Can you work these out from the drawing? Everything is in mm from the part's minimum corner. Give positions to 0.01 mm unless a question says otherwise; leave off trailing zeros. Loops run counter-clockwise (first coordinate to the right, second up) from the corner with the lowest first, then second, coordinate; pieces in that order, holes last. Notation, with made-up numbers: (-10.5, 60) - (9.5, 60) arc R30 cw to (9.5, 87) - close; hole circle Ø10 at (4, -7). An arc over 180 degrees is marked (long way). Answer in a Markdown table with one row per item.
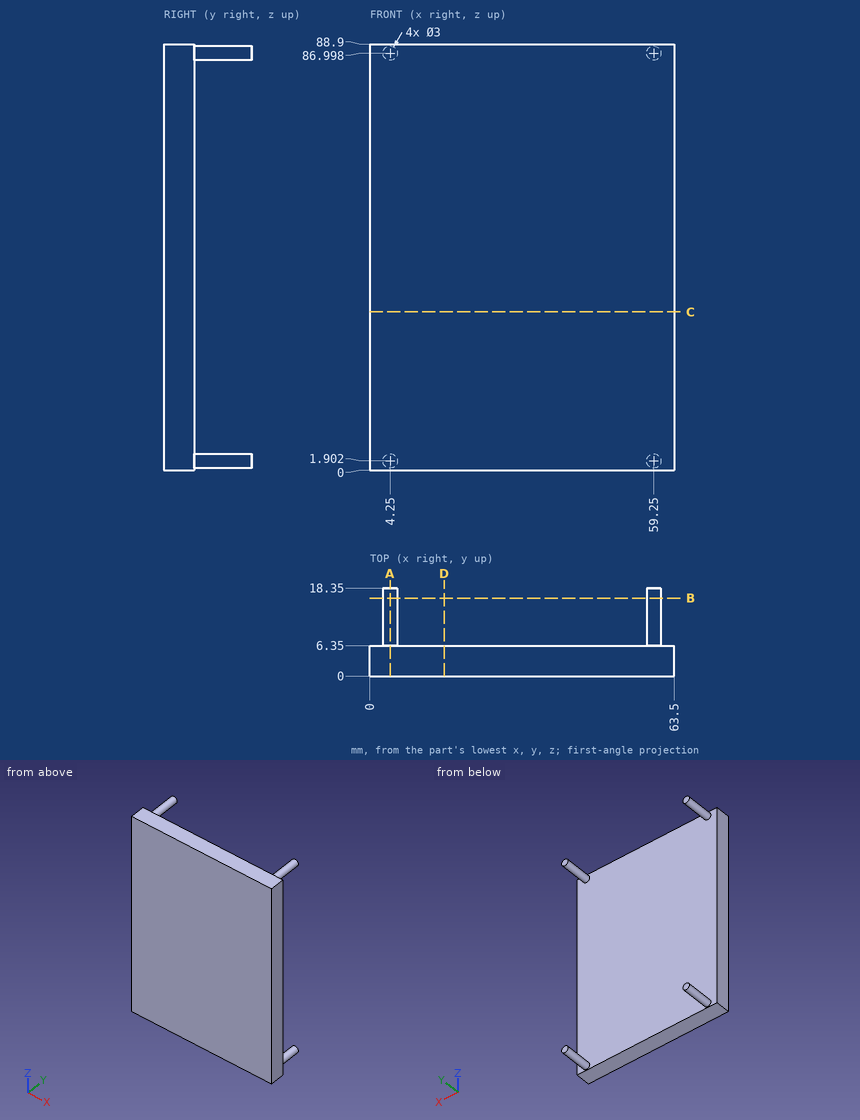
Q1. Imagine slicing it at C-C, the plane z = 33. Write out the boundary of the cut face in (x, y).
Checked values:
| item | result |
|---|---|
| outline | (0, 0) - (63.5, 0) - (63.5, 6.35) - (0, 6.35) - close |
Q2. Imagine slicing it at B-B, the plane y = 16.25. Write out the boundary of the cut face in (x, z).
Checked values:
| item | result |
|---|---|
| outline | circle Ø3 at (4.25, 1.9); circle Ø3 at (4.25, 87); circle Ø3 at (59.25, 1.9); circle Ø3 at (59.25, 87) |
Q3. Imagine slicing it at D-D, the plane x = 15.5. Write out the boundary of the cut face in (y, z).
Checked values:
| item | result |
|---|---|
| outline | (0, 0) - (6.35, 0) - (6.35, 88.9) - (0, 88.9) - close |
Q4. For pin 1 (10 mm diameter, centred on x = 50, y = 7, fed in from +Z); pin 2 (19 mm diameter, centred on x = 36.5, z = 30, fed in from +Y); pin 3 (3 mm diameter, centred on x = 46.5, y = 9.5, fed in from +Z) (3 decimals), each with a flat end and sliding along its axis, tell me the tip position at first contact or that it passes through.
Checked values:
| item | result |
|---|---|
| pin 1 | stops at z = 88.9 |
| pin 2 | stops at y = 6.35 |
| pin 3 | passes through |
Q5. If I drill on line 1 (Y direction, x = 37.5, z = 58.5), over which ranges is the centre line in solid material (lowest first)? Write a range as [from, to].
Checked values:
| item | result |
|---|---|
| line 1 | y = [0, 6.35] |
Q6. Imagine slicing it at A-A, the plane x = 4.25. Write out the boundary of the cut face in (y, z).
Checked values:
| item | result |
|---|---|
| outline | (0, 0) - (6.35, 0) - (6.35, 0.4) - (18.35, 0.4) - (18.35, 3.4) - (6.35, 3.4) - (6.35, 85.5) - (18.35, 85.5) - (18.35, 88.5) - (6.35, 88.5) - (6.35, 88.9) - (0, 88.9) - close |
